Build history of the part. All positions in model axes, mm. Give positions to 0.01 mm unless a question says otherwise; leave off trailing zeros. Write each loop counter-clockwise with the first axis right and the second up, starting at its lowest first coordinate (ties: lowest second). Pieces come first, ordered by that corner, then holes. Notation, with made-up numbers: (-15.5, -10.75) -> (-0.5, -10.75) arc R21 cw to (-0.5, 28.25) -> close; hole circle Ø10 at (34.5, -13.75). An arc over 180 degrees is marked (long way). Put each result on its own line as item: value. Start each with the question number.
Item 1: Slice it at C-C, the plane x = -1891.5. List the corners of the cut face in (y, z).
Item 2: Drill centre lines: line 1 along Y through (x, z) = (-1914.5, 217.5); line 2 along Z through (x, y) = (-1929.5, -11); line 3 along Z through (x, y) = (-1909.5, -5). Where is each one in solid material? Low to high.
Item 3: Flat gauge pins, fed straight in: pin 1 Ø13 at (x, z) = (-1928.2, 516.07) entering from -Y; pin 2 Ø12 at (x, z) = (-1909, 420) entering from +Y; pin 3 Ø5 at (y, z) = (-20.5, -203.5) entering from +X; pin 4 Ø2 at (y, z) = (-20, -128.5) entering from +X. Where does each tip first touch, or does it go through?
Item 4: Slice it at B-B, the plane z = -478. List the corners of the cut face in (x, y), plus the area to 3 significant figures.
Item 5: Slice it at A-A, the plane y = -28. List the corners of the cut face in (x, z).
```python
from build123d import *

# Parameters (mm, degrees)
F0_W        = 88.9
F0_H        = 1140
F0_R        = 5
F1_DEPTH    = 38.1
F2_T1_DEPTH = 1382.8162885805
F2_T3_DEPTH = 331.7162885805


# Not quite as in the source:
# - a fillet or chamfer that OpenCascade refuses, or shapes differently, is made with other operations: its cross-section is extruded or revolved along the edge and cut away or added


with BuildPart() as f1:
    # F0 (on Front) → F1 (new body)
    with BuildSketch(Plane.XZ):
        with Locations((-1911.2522443051, 3.6825537682)):
            Rectangle(F0_W, F0_H)
        with Locations((-1928.2022443051, 516.0674452782)):
            Circle(F0_R, mode=Mode.SUBTRACT)
    extrude(amount=F1_DEPTH)

    # F2: fillet of radius 50 on 2 edges, made by hand

    # F2_s2 → F2_t1 (cut)
    with BuildSketch(Plane.XY.offset(-687.7255905221)):
        with BuildLine():
            ThreePointArc((-1866.8022443051, -38.1), (-1884.5029032971, -10.6617234745), (-1915.3655020212, 0))
            Line((-1915.3655020212, 0), (-1866.8022443051, 0))
            Line((-1866.8022443051, 0), (-1866.8022443051, -38.1))
        make_face()
    extrude(amount=F2_T1_DEPTH, mode=Mode.SUBTRACT)

    # F2_s4 → F2_t3 (cut)
    with BuildSketch(Plane.YZ.offset(-2077.1103885953)):
        with BuildLine():
            ThreePointArc((-38.1, 573.6825537682), (-10.6617234745, 555.9818947761), (0, 525.1192960521))
            Line((0, 525.1192960521), (0, 573.6825537682))
            Line((0, 573.6825537682), (-38.1, 573.6825537682))
        make_face()
    extrude(amount=F2_T3_DEPTH, mode=Mode.SUBTRACT)


solid = f1.part
```
Values follow:
1. outline: (-38.1, -566.32) -> (-6.06, -566.32) -> (-6.06, 548.98) arc R50 ccw to (-38.1, 573.68) -> close
2. line 1: -38.1 to -0.01
2. line 2: -566.32 to 511.24, 520.9 to 556.41
2. line 3: -566.32 to 546.91
3. pin 1: y = -38.1
3. pin 2: y = 0
3. pin 3: x = -1873.28
3. pin 4: x = -1874.63
4. outline: (-1955.7, -38.1) -> (-1866.8, -38.1) arc R50 ccw to (-1915.37, 0) -> (-1955.7, 0) -> close
4. area: 2,910 mm2
5. outline: (-1955.7, -566.32) -> (-1870.47, -566.32) -> (-1870.47, 570.02) -> (-1955.7, 570.02) -> close; hole circle Ø10 at (-1928.2, 516.07)
